```python
from build123d import *

# Parameters (mm, degrees)
F0_W        = 15
F0_H        = 27
F0_W_2      = 13
F0_H_2      = 24
F1_DEPTH    = 1.2
F2_DEPTH    = 4
F3_R        = 2
F4_W        = 2.6
F4_H        = 17
F4_W_2      = 0.4
F5_DEPTH    = 1.5
F6_T1_DEPTH = 21
F6_T3_DEPTH = 22
F7_T4_DEPTH = 22.1433659759
F8_R        = 0.75


# Not quite as in the source:
# - a fillet or chamfer that OpenCascade refuses, or shapes differently, is made with other operations: its cross-section is extruded or revolved along the edge and cut away or added


with BuildPart() as f1:
    # F0 (on Top) → F1 (new body)
    with BuildSketch(Plane.XY):
        Rectangle(F0_W, F0_H)
        Rectangle(F0_W_2, F0_H_2, mode=Mode.SUBTRACT)
    extrude(amount=F1_DEPTH)

    # F0 (on Top) → F2 (join)
    with BuildSketch(Plane.XY):
        Rectangle(F0_W_2, F0_H_2)
    extrude(amount=F2_DEPTH)

    # F3
    f3_edges = [f1.edges().sort_by_distance(p)[0] for p in [
        (6.5, 12, 2.6),
        (7.5, 13.5, 0.6),
        (-6.5, 12, 2.6),
        (-7.5, 13.5, 0.6),
        (-6.5, -12, 2.6),
        (-7.5, -13.5, 0.6),
        (7.5, -13.5, 0.6),
        (6.5, -12, 2.6),
    ]]
    fillet(f3_edges, radius=F3_R)

    # F4 (on face) → F5 (join)
    with BuildSketch(Plane.XY.offset(4)):
        with Locations((-5.2, 0)):
            Rectangle(F4_W, F4_H)
        with Locations((6.7, 0)):
            Rectangle(F4_W_2, F4_H)
        with Locations((5.2, 0)):
            Rectangle(F4_W, F4_H)
        with Locations((-6.7, 0)):
            Rectangle(F4_W_2, F4_H)
    extrude(amount=F5_DEPTH)

    # F6: fillet of radius 1 on 4 edges, made by hand

    # F6_s2 → F6_t1 (cut)
    with BuildSketch(Plane.XZ.offset(-10.5)):
        with BuildLine():
            ThreePointArc((6.5, 4), (6.794427191, 4.3527864045), (6.9, 4.8))
            Line((6.9, 4.8), (6.9, 4))
            Line((6.9, 4), (6.5, 4))
        make_face()
    extrude(amount=F6_T1_DEPTH, mode=Mode.SUBTRACT)

    # F6_s4 → F6_t3 (cut)
    with BuildSketch(Plane.XZ.offset(-11)):
        with BuildLine():
            ThreePointArc((6.9, 4.5), (6.6071067812, 5.2071067812), (5.9, 5.5))
            Line((5.9, 5.5), (6.9, 5.5))
            Line((6.9, 5.5), (6.9, 4.5))
        make_face()
        with BuildLine():
            ThreePointArc((-3.9, 4.5), (-4.1928932188, 5.2071067812), (-4.9, 5.5))
            Line((-4.9, 5.5), (-3.9, 5.5))
            Line((-3.9, 5.5), (-3.9, 4.5))
        make_face()
        with BuildLine():
            ThreePointArc((3.9, 4.5), (4.1928932188, 5.2071067812), (4.9, 5.5))
            Line((4.9, 5.5), (3.9, 5.5))
            Line((3.9, 5.5), (3.9, 4.5))
        make_face()
    extrude(amount=F6_T3_DEPTH, mode=Mode.SUBTRACT)

    # F7: chamfer of 1 on 1 edges, made by hand


with BuildPart() as f7_tool2:
    # F7_s3 → F7_t4 (new body)
    with BuildSketch(Plane.XZ.offset(-11.071682988)):
        Polygon((-5.9, 4), (-6.9, 5), (-6.9, 4), align=None)
    extrude(amount=F7_T4_DEPTH)

    split(bisect_by=Plane.YZ.offset(-6.5), keep=Keep.BOTTOM)


with BuildPart() as f1_1:
    add(f1.part)

    # F7_t1: cut F7_tool2
    add(f7_tool2.part, mode=Mode.SUBTRACT)

    # F8
    f8_edges = [f1_1.edges().sort_by_distance(p)[0] for p in [
        (6.888686, 0, 4.65),
    ]]
    fillet(f8_edges, radius=F8_R)


solid = f1_1.part
```
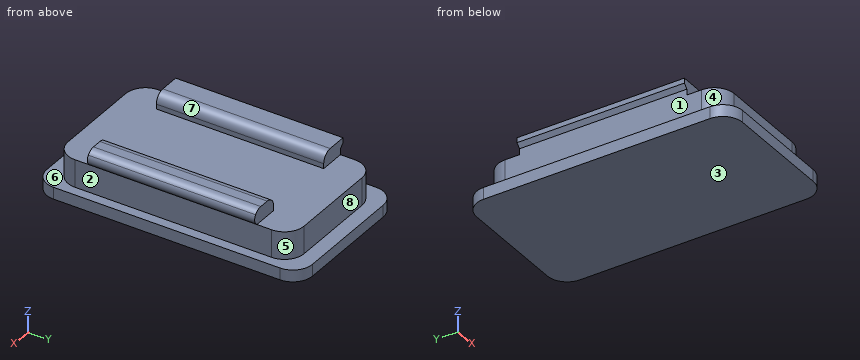
For this review, take the finished solid that the model builds, in its own axes (mm). Face numbers are marked on the shaded views. A direction names the side the tool comes from. Round coordinates to 2 decimals unless told otherwise and drop trailing zeros. Write each loop counter-clockwise with the first axis right and the second up, starting at its lowest first coordinate (ties: lowest second). Pieces come first, ordered by that corner, then holes. Notation, with made-up numbers: (62, 65.25) -> (68, 65.25) arc R25 ccw to (68, 101.25) -> close; hole circle Ø4 at (75.25, 7.5). An arc over 180 degrees is marked (long way). One line per question, with ' | ' between items. Start each with the question number.
1) Wall thickness on line 1 along Z through (x, y) = (3, -4.75); line 2 along Y through (x, z) = (-6, 4.7); line 3 along X through (y, z) = (-8, 3.5): over which ranges is each line inside the solid? List them lowest first.
2) Mouldability with a two-part tool opening along Z and no side actions: class the marked faces 1, 2, 3 and 4 as +Z half, -Z half, draft (parallel to the pull), parting line (faces both ways), or undercut.
3) Machinability: for the marked faces 5, 6, 7 and 8, which of the approach directions +Z, -Z, +X, -X, +Y, -Y give a long, thin tool a straight path to every point of the face, cutting with its end or side? Answer none if there is none.
4) Add section A-A (x = 0.25). Write out the cut boundary in (y, z), and give its area (3 significant figures).
5) Add section B-B (z = 2.6). Write out the cut boundary in (x, y).
6) For pin 1 Ø0.8 at (x, z) = (-5.5, 4.5) entering from -Y; pin 2 Ø1.4 at (x, z) = (1, 3) entering from -Y; pin 3 Ø0.6 at (y, z) = (-2.5, 4) entering from +X, all flat-tipped, find the tip position at first contact; note any pin that passes through.
Reported:
1) line 1: z = 0 to 4 | line 2: y = -8.5 to 8.5 | line 3: x = -6.5 to 6.5
2) face 1: undercut | face 2: undercut | face 3: -Z half | face 4: draft
3) face 5: +Z, +X, +Y | face 6: none | face 7: +Z, +Y, -Y | face 8: +Z, +X, -X, +Y
4) outline: (-13.5, 0) -> (13.5, 0) -> (13.5, 1.2) -> (12, 1.2) -> (12, 4) -> (-12, 4) -> (-12, 1.2) -> (-13.5, 1.2) -> close | area: 99.6 mm²
5) outline: (-6.5, -10) arc R2 ccw to (-4.5, -12) -> (4.5, -12) arc R2 ccw to (6.5, -10) -> (6.5, 10) arc R2 ccw to (4.5, 12) -> (-4.5, 12) arc R2 ccw to (-6.5, 10) -> close
6) pin 1: stops at y = -8.5 | pin 2: stops at y = -12 | pin 3: stops at x = 6.76
